from build123d import *

# Parameters (mm, degrees)
F0_W     = 25.4
F0_H     = 17.526
F1_DEPTH = 2.54
F2_W     = 25.4
F2_H     = 4.318
F2_R     = 2.54
F3_DEPTH = 3.81
F4_W     = 1.143
F4_H     = 4.318
F4_R     = 1.27
F5_DEPTH = 2.54


with BuildPart() as f1:
    # F0 (on Top) → F1 (new body)
    with BuildSketch(Plane.XY):
        Rectangle(F0_W, F0_H)
    extrude(amount=F1_DEPTH)

    # F2 (on face) → F3 (join)
    with BuildSketch(Plane.XY.offset(2.54)):
        with Locations((0, 6.604)):
            Rectangle(F2_W, F2_H)
        with Locations((-8.763, -3.937)):
            Circle(F2_R)
        with Locations((8.763, -3.937)):
            Circle(F2_R)
    extrude(amount=F3_DEPTH)

    # F4 (on face) → F5 (join)
    with BuildSketch(Plane.XY.offset(6.35)):
        with Locations((-12.1285, 6.604)):
            Rectangle(F4_W, F4_H)
        with Locations((12.1285, 6.604)):
            Rectangle(F4_W, F4_H)
        with Locations((-8.763, -3.937)):
            Circle(F4_R)
        with Locations((8.763, -3.937)):
            Circle(F4_R)
    extrude(amount=F5_DEPTH)


solid = f1.part
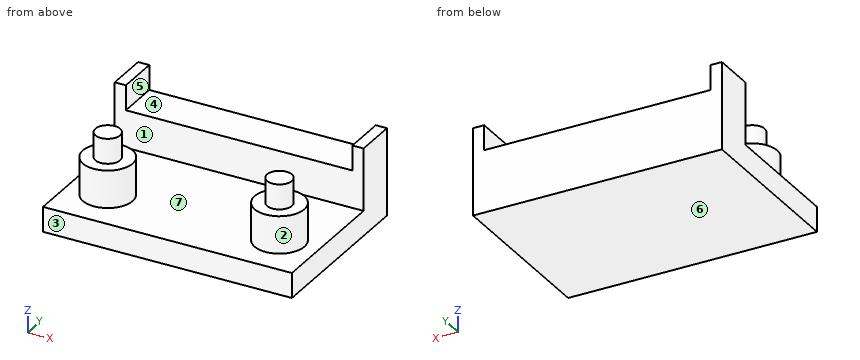
For this review, take the finished solid that the model builds, in its own axes (mm). Face numbers are marked on the shaded views. A direction names the side the tool comes from. Give positions to 0.01 mm unless a question says otherwise; leave off trailing zeros. Write each loop counter-clockwise with the first axis right and the second up, starting at its lowest first coordinate (ties: lowest second). Pieces come first, ordered by that corner, then holes. Notation, with made-up numbers: (59.5, 73) -> (71.5, 73) arc R18 ccw to (71.5, 104) -> close; hole circle Ø8 at (12.25, -18.5). An arc over 180 degrees is marked (long way). Use CSV: the item, a comma, the result in double quotes.
Q1. Tool access review of the marked faces 5, 6 and 7: name each direction out of +Z, -Z, +X, -X, +Y, -Y from which nothing blocks a thin tool from reaching the whole face with its end or side.
Conclusion:
face 5,"+Z, +Y, -Y"
face 6,"-Z, +X, -X, +Y, -Y"
face 7,"+Z"
Q2. For P1, Ø4, axis at x = -0.5, y = -1.5, coming from the +Z side; P2, Ø1.5, axis at x = -7, z = 4.5, coming from the -Y side; P3, Ø4.5, axis at x = -1.5, y = 7, coming from the +Z side, all flat-tipped, find the tip position at first contact; note any pin that passes through.
Conclusion:
P1,"z = 2.54"
P2,"y = -6.27"
P3,"z = 6.35"
Q3. Take a section at B-B, the plane y = 5. Write out the cut boundary in (x, z).
Conclusion:
outline,"(-12.7, 0) -> (12.7, 0) -> (12.7, 8.89) -> (11.56, 8.89) -> (11.56, 6.35) -> (-11.56, 6.35) -> (-11.56, 8.89) -> (-12.7, 8.89) -> close"
Q4. Take a section at C-C, the plane z = 3.5. Write out the cut boundary in (x, y) (3 decimals).
Conclusion:
outline,"(-12.7, 4.445) -> (12.7, 4.445) -> (12.7, 8.763) -> (-12.7, 8.763) -> close; circle Ø5.08 at (-8.763, -3.937); circle Ø5.08 at (8.763, -3.937)"
Q5. Mouldability with a two-part tool opening along Y and no side actions: class the marked faces 1, 2, 3 and 4 as pulls with the +Y half, pulls with the -Y half, needs draft (parallel to the pull), parting line crosses it, or undercut.
Conclusion:
face 1,"undercut"
face 2,"undercut"
face 3,"pulls with the -Y half"
face 4,"needs draft"
Q6. To check wall thickness, follow probe 1 along X at (y, z) = (-3.75, 3); probe 2 along Z at (x, y) = (11.5, -5.75); probe 3 along X at (y, z) = (7.5, 8). State the ranges of each line that lie inside material, in increasing order. Write a range as [from, to].
Conclusion:
probe 1,"[-11.3, -6.23], [6.23, 11.3]"
probe 2,"[0, 2.54]"
probe 3,"[-12.7, -11.56], [11.56, 12.7]"
Q7. Take a section at A-A, the plane z = 7. Write out the cut boundary in (x, y) (3 decimals), then the cut area to 3 significant figures.
Conclusion:
outline,"(-12.7, 4.445) -> (-11.557, 4.445) -> (-11.557, 8.763) -> (-12.7, 8.763) -> close; circle Ø2.54 at (-8.763, -3.937); circle Ø2.54 at (8.763, -3.937); (11.557, 4.445) -> (12.7, 4.445) -> (12.7, 8.763) -> (11.557, 8.763) -> close"
area,"20.0 mm2"
Q8. Take a section at D-D, the plane x = -2.25. Write out the cut boundary in (y, z) (3 decimals), then the cut area to 3 significant figures.
Conclusion:
outline,"(-8.763, 0) -> (8.763, 0) -> (8.763, 6.35) -> (4.445, 6.35) -> (4.445, 2.54) -> (-8.763, 2.54) -> close"
area,"61.0 mm2"
